```python
from build123d import *

# Parameters (mm, degrees)
SKETCH1_W           = 15
SKETCH1_H           = 18
BOSS_EXTRUDE1_DEPTH = 7
CUT_EXTRUDE1_DEPTH  = 14.2
SKETCH8_W           = 0.5
SKETCH8_H           = 2.6
CUT_EXTRUDE4_DEPTH  = 10
SKETCH9_W           = 16
SKETCH9_H           = 6
BOSS_EXTRUDE2_DEPTH = 18
SKETCH13_W          = 16
SKETCH13_H          = 6
BOSS_EXTRUDE3_DEPTH = 18
SKETCH14_W          = 15
SKETCH14_H          = 3
CUT_EXTRUDE5_DEPTH  = 32.55
FILLET1_R           = 0.5


with BuildPart() as part:
    # Sketch1 → Boss-Extrude1 (new body)
    with BuildSketch(Plane(origin=(0, 0, 0), x_dir=(1, 0, 0), z_dir=(0, 1, 0))):
        Rectangle(SKETCH1_W, SKETCH1_H)
    extrude(amount=BOSS_EXTRUDE1_DEPTH)

    # Sketch2 → Cut-Extrude1 (cut)
    with BuildSketch(Plane.XY.offset(9)):
        Polygon((-4.675, 2.6), (-4.675, 0), (-1.1, 0), (-1.1, 2.6), (-0.6, 2.6), (-0.6, 0), (0.6, 0), (0.6, 2.6), (1.1, 2.6), (1.1, 0), (4.675, 0), (4.675, 2.6), (6.85, 2.6), (6.85, 4), (-6.85, 4), (-6.85, 2.6), align=None)
    extrude(amount=-CUT_EXTRUDE1_DEPTH, mode=Mode.SUBTRACT)

    # Sketch8 → Cut-Extrude4 (cut)
    with BuildSketch(Plane.XY.offset(9)):
        with Locations((-0.85, 1.3)):
            Rectangle(SKETCH8_W, SKETCH8_H)
        with Locations((0.85, 1.3)):
            Rectangle(SKETCH8_W, SKETCH8_H)
    extrude(amount=-CUT_EXTRUDE4_DEPTH, mode=Mode.SUBTRACT)

    # Sketch9 → Boss-Extrude2 (add)
    with BuildSketch(Plane.ZY.offset(7.5)):
        with Locations((0, 3)):
            Rectangle(SKETCH9_W, SKETCH9_H)
    extrude(amount=BOSS_EXTRUDE2_DEPTH)

    # Sketch13 → Boss-Extrude3 (add)
    with BuildSketch(Plane(origin=(7.5, 0, 0), x_dir=(0, 0, -1), z_dir=(1, 0, 0))):
        with Locations((0, 3)):
            Rectangle(SKETCH13_W, SKETCH13_H)
    extrude(amount=BOSS_EXTRUDE3_DEPTH)

    # Sketch14 → Cut-Extrude5 (cut)
    with BuildSketch(Plane.XY.offset(9)):
        with Locations((16.5, 4.5)):
            Rectangle(SKETCH14_W, SKETCH14_H)
        with Locations((-16.5, 4.5)):
            Rectangle(SKETCH14_W, SKETCH14_H)
    extrude(amount=-CUT_EXTRUDE5_DEPTH, mode=Mode.SUBTRACT)

    # Fillet1
    fillet1_edges = [part.edges().sort_by_distance(p)[0] for p in [
        (-7.5, 0, 8.5),
        (-25.5, 6, 0),
        (7.5, 0, -8.5),
        (25.5, 6, 0),
        (-7.5, 7, 0),
        (9, 6, 0),
        (-9, 6, 0),
        (6.0875, 0, 9),
        (0, 7, 9),
        (4.675, 0, 1.9),
        (-4.675, 0, 1.9),
        (7.5, 7, 0),
        (-6.0875, 0, 9),
        (-7.5, 0, -8.5),
        (0, 0, -9),
        (7.5, 0, 8.5),
        (7.5, 3.5, 9),
        (-7.5, 3.5, 9),
        (-7.5, 3.5, -9),
        (7.5, 3.5, -9),
        (0, 7, -9),
    ]]
    fillet(fillet1_edges, radius=FILLET1_R)


solid = part.part
```
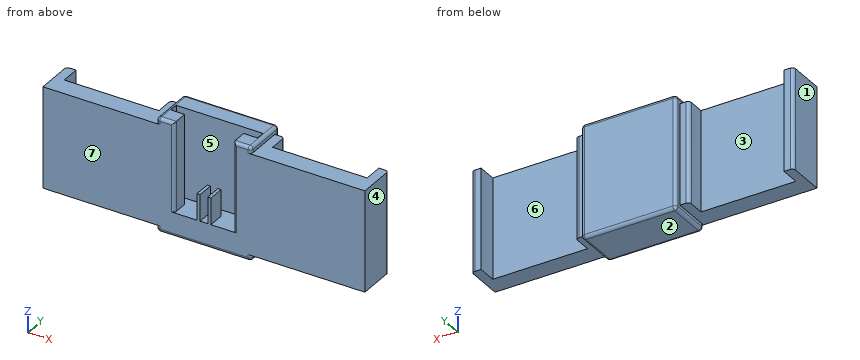
Input: part model. Units: mm. Frame: model coordinates. Face numbers are marked on the shaded views. A direction names the side the tool comes from. Round coordinates to 2 decimals unless told otherwise and drop trailing zeros. Loops run counter-clockwise (first coordinate to the right, second up) from the corner with the lowest first, then second, coordinate; pieces in that order, holes last. Notation, with made-up numbers: M 76,50 L 93,50 A23 ccw 93,73 Z; hole C 76.5,-31.75 d8. An arc over 180 degrees is marked long. Answer in a Markdown table with one row per item. Add a question column.
1. Mould query, pull axis X, two halves, no side actions, for the marked faces 1, 2, 3 and 4. Classes: released by +X, released by -X, zero draft, split by the parting line, or undercut.
2. Section A-A (y = 3.5). Output: boundary loops of the cut face in (x, z).
3. Set-up query: the marked faces 5, 6 and 7. Return all of +Z, -Z, +X, -X, +Y, -Y with unobstructed straight access to the full face (end or side cutting, diameter ignored); none if empty.
4. Ray query, probe 1 along X at (y, z) = (5.25, -1); probe 2 along X at (y, z) = (3.25, -0.5); probe 3 along Y at (x, z) = (-6.5, -0.75). Return the intervals inside material, ascending.
5. Section D-D (y = 1.25). Output: boundary loops of the cut face in (x, z) (3 decimals), and give its area (3 significant figures).
6. Contact query for flat-ended pins moving along their axis: pin 1 (1.2 mm diameter, centred on x = -2, y = 2.5, fed in from +Z); pin 2 (1.1 mm diameter, centred on x = -24.5, z = -4, fed in from +Y); pin 3 (2 mm diameter, centred on x = -14, y = 2, fed in from -Z). Output: stop coordinate, or through.
7. Section B-B (x = 2). Output: boundary loops of the cut face in (y, z), and give its area (3 significant figures).
Values follow:
| question | item | result |
|---|---|---|
| 1 | face 1 | released by -X |
| 1 | face 2 | zero draft |
| 1 | face 3 | undercut |
| 1 | face 4 | released by +X |
| 2 | outline | M -25.5,-8 L -24,-8 L -24,8 L -25.5,8 Z; M -9,-8 L -7.5,-8 L -7.5,-8.5 A0.5 ccw -7,-9 L 7,-9 A0.5 ccw 7.5,-8.5 L 7.5,-8 L 9,-8 L 9,8 L 7.5,8 L 7.5,8.5 A0.5 ccw 7,9 L 6.85,9 L 6.85,-5.2 L -6.85,-5.2 L -6.85,9 L -7,9 A0.5 ccw -7.5,8.5 L -7.5,8 L -9,8 Z; M 24,-8 L 25.5,-8 L 25.5,8 L 24,8 Z |
| 3 | face 5 | +Z |
| 3 | face 6 | +Z, -Z, +Y |
| 3 | face 7 | +Z, -Z, +X, -X, -Y |
| 4 | probe 1 | -25.5 to -24, -9 to 9, 24 to 25.5 |
| 4 | probe 2 | -25.5 to -24, -9 to -6.85, 6.85 to 9, 24 to 25.5 |
| 4 | probe 3 | 0 to 2.6, 4 to 7 |
| 5 | outline | M -25.5,-8 L -7.5,-8 L -7.5,-8.5 A0.5 ccw -7,-9 L 7,-9 A0.5 ccw 7.5,-8.5 L 7.5,-8 L 25.5,-8 L 25.5,8 L 7.5,8 L 7.5,8.5 A0.5 ccw 7,9 L 4.675,9 L 4.675,-5.2 L 1.1,-5.2 L 1.1,-1 L 0.6,-1 L 0.6,-5.2 L -0.6,-5.2 L -0.6,-1 L -1.1,-1 L -1.1,-5.2 L -4.675,-5.2 L -4.675,9 L -7,9 A0.5 ccw -7.5,8.5 L -7.5,8 L -25.5,8 Z |
| 5 | area | 717 mm^2 |
| 6 | pin 1 | z = -5.2 |
| 6 | pin 2 | y = 6 |
| 6 | pin 3 | z = -8 |
| 7 | outline | M 0,-8.5 A0.5 ccw 0.5,-9 L 6.5,-9 A0.5 ccw 7,-8.5 L 7,8.5 A0.5 ccw 6.5,9 L 4,9 L 4,-5.2 L 0,-5.2 Z |
| 7 | area | 69.0 mm^2 |
